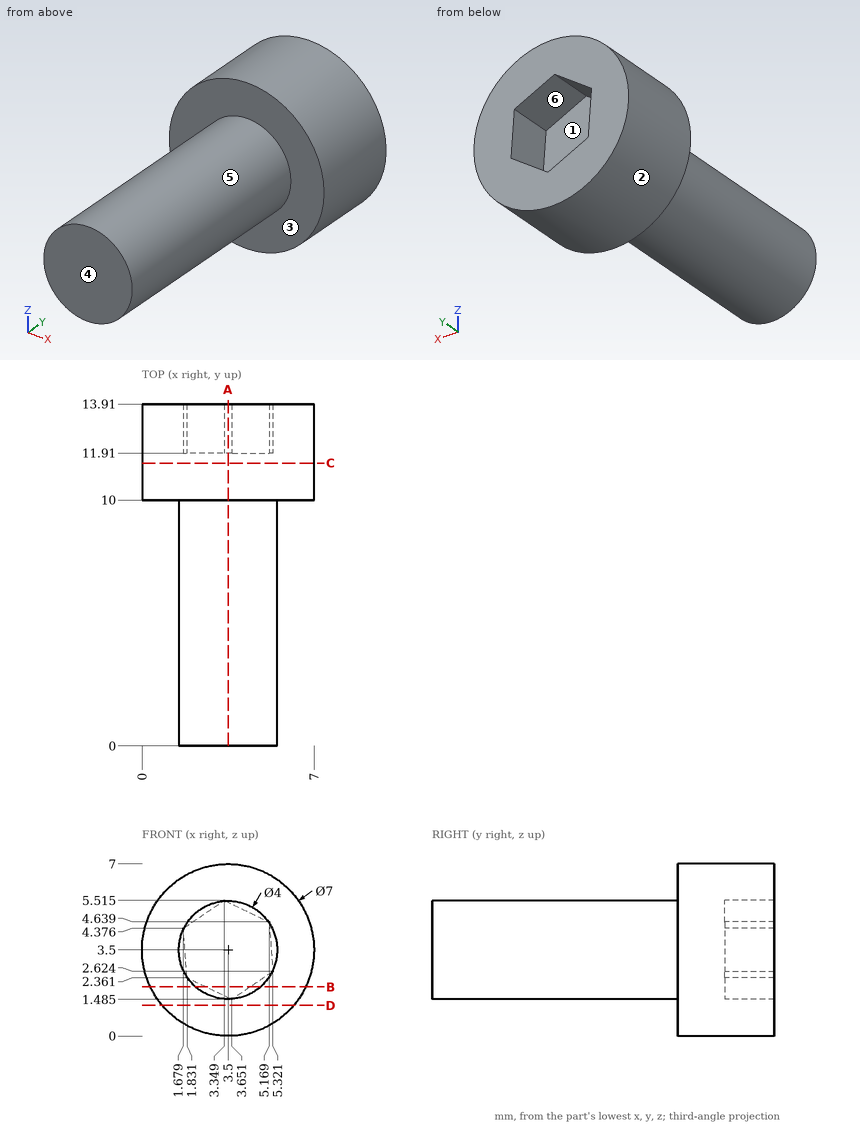
Verification items for this drawing (mm, ordinates from the low corner). A direction names the side the tool comes from. Coordinates: 2 decimals unless noted, no trailing zeros. Order: outer loops, then holes, each group sorted by start corner. A loop starts at its lowest first (then second) coordinate and runs counter-clockwise, first axis right, second up.
Q1. Thickness scan on probe 1 along Y at (x, z) = (4.5, 3.75); probe 2 along Y at (x, z) = (6, 5); probe 3 along X at (y, z) = (12.5, 2.5) (1 decimal). Record the ranges inside material, lowest first.
Reply:
probe 1: y = 0 to 11.91
probe 2: y = 10 to 13.91
probe 3: x = 0.1 to 1.8, 5.1 to 6.9
Q2. Sectioned sample at A-A on x = 3.5. Record the cut outline in (y, z).
Reply:
outline: (0, 1.5) - (10, 1.5) - (10, 0) - (13.91, 0) - (13.91, 1.56) - (11.91, 1.56) - (11.91, 5.44) - (13.91, 5.44) - (13.91, 7) - (10, 7) - (10, 5.5) - (0, 5.5) - close
Q3. Draft check along Z on the marked faces 4, 5 and 6. Enter one of: released by +Z, released by -Z, zero draft, split by the parting line, or undercut.
Reply:
face 4: zero draft
face 5: split by the parting line
face 6: undercut
Q4. Sectioned sample at D-D on z = 1.25. Record the cut outline in (x, y).
Reply:
outline: (0.82, 10) - (6.18, 10) - (6.18, 13.91) - (0.82, 13.91) - close
Q5. Sectioned sample at C-C on y = 11.5. Record the cut outline in (x, z), and give its area (3 significant figures).
Reply:
outline: circle Ø7 at (3.5, 3.5)
area: 38.5 mm2
Q6. Sectioned sample at B-B on z = 2. Record the cut outline in (x, y).
Reply:
outline: (0.34, 10) - (2.18, 10) - (2.18, 0) - (4.82, 0) - (4.82, 10) - (6.66, 10) - (6.66, 13.91) - (4.41, 13.91) - (4.41, 11.91) - (2.58, 11.91) - (2.58, 13.91) - (0.34, 13.91) - close
Q7. Depth check by flat-ended pin: pin 1 Ø4 at (y, z) = (5, 4.5) entering from +X; pin 2 Ø2 at (x, y) = (1.5, 3.5) entering from +Z; pin 3 Ø1.8 at (x, z) = (3, 3.5) entering from +Y. Enter the tip coordinate at first touch or a pass-through.
Reply:
pin 1: stops at x = 5.5
pin 2: stops at z = 5.23
pin 3: stops at y = 11.91
Q8. Tool access check on the marked faces 1, 2 and 3. Record the directions out of +Z, -Z, +X, -X, +Y, -Y that give a thin tool (end or side, any length) a straight path to the whole face; none if there is none.
Reply:
face 1: +Y
face 2: +Y, -Y
face 3: -Y
